```python
from build123d import *
from OCP.BRepFilletAPI import BRepFilletAPI_MakeChamfer

# Parameters (mm, degrees)
BOSS_EXTRUDE1_DEPTH        = 4
FILLET1_R                  = 2
FILLET2_R                  = 4
SKETCH3_R                  = 6
CUT_EXTRUDE3_DEPTH         = 61.942595941
SKETCH4_R                  = 1.75
CUT_EXTRUDE6_DEPTH         = 61.942595941
CUT_EXTRUDE7_DEPTH         = 10
CUT_EXTRUDE8_START         = -12.533
CUT_EXTRUDE8_DEPTH         = 25.3653
CHAMFER1_SIZE              = 2
CHAMFER1_SIZE_2            = 0.932615316
CHAMFER1_OF_MIRROR1_SIZE   = 0.932615316
CHAMFER1_OF_MIRROR1_SIZE_2 = 2
CHAMFER2_SIZE              = 0.5


with BuildPart() as part:
    # Sketch1 → Boss-Extrude1 (new body)
    with BuildSketch(Plane.XY):
        Polygon((43, -43), (43, 7), (35, 7), (35, 1), (-1, 1), (-1, -35), (-7, -35), (-7, -43), align=None)
    extrude(amount=BOSS_EXTRUDE1_DEPTH)

    # Fillet1
    fillet1_edges = [part.edges().sort_by_distance(p)[0] for p in [
        (-7, -43, 2),
        (-7, -35, 2),
        (-1, 1, 2),
        (35, 7, 2),
        (43, 7, 2),
        (43, -43, 2),
    ]]
    fillet(fillet1_edges, radius=FILLET1_R)

    # Fillet2
    fillet2_edges = [part.edges().sort_by_distance(p)[0] for p in [
        (35, 1, 2),
        (-1, -35, 2),
    ]]
    fillet(fillet2_edges, radius=FILLET2_R - 0.0001)  # a hair under: the kernel refuses the full size

    # Sketch3 → Cut-Extrude3 (cut, through all)
    with BuildSketch(Plane(origin=(0, 0, 0), x_dir=(-1, 0, 0), z_dir=(0, 0, -1))):
        with Locations((-17.899660586, -17.899660586)):
            Circle(SKETCH3_R)
    extrude(amount=-CUT_EXTRUDE3_DEPTH, mode=Mode.SUBTRACT)

    # Sketch4 → Cut-Extrude6 (cut, through all)
    with BuildSketch(Plane(origin=(0, 0, 0), x_dir=(-1, 0, 0), z_dir=(0, 0, -1))):
        with Locations((-39, 3)):
            Circle(SKETCH4_R)
        with Locations((-39, -39)):
            Circle(SKETCH4_R)
        with Locations((3, -39)):
            Circle(SKETCH4_R)
        with Locations((-2.025269256, -2.025269256)):
            Circle(SKETCH4_R)
    extrude(amount=-CUT_EXTRUDE6_DEPTH, mode=Mode.SUBTRACT)

    # Sketch5 → Cut-Extrude7 (cut, symmetric)
    with BuildSketch(Plane.ZY.offset(-17.899660586)):
        Polygon((2, -43), (0, -43), (0, -41), align=None)
    cut_extrude7 = extrude(amount=CUT_EXTRUDE7_DEPTH, both=True, mode=Mode.SUBTRACT)

    # Sketch6 → Cut-Extrude8 (cut)
    with BuildSketch(Plane.ZY.offset(-17.899660586).offset(CUT_EXTRUDE8_START)):
        Polygon((0, 1), (0, -1), (1.5, -1), (3.5, 1), align=None)
    cut_extrude8 = extrude(amount=CUT_EXTRUDE8_DEPTH, mode=Mode.SUBTRACT)

    # Chamfer1
    chamfer1_edges_1 = [part.edges().sort_by_distance(p)[0] for p in [
        (5.067360586, -1, 0.75),
    ]]
    chamfer1_side_1 = [part.faces().sort_by_distance(p)[0] for p in [
        (5.067360586, -0.981347694, 0.75),
    ]]
    chamfer1_edges_2 = [part.edges().sort_by_distance(p)[0] for p in [
        (30.432660586, -1, 0.75),
    ]]
    chamfer1_side_2 = [part.faces().sort_by_distance(p)[0] for p in [
        (30.41400828, -1, 0.75),
    ]]
    chamfer1 = BRepFilletAPI_MakeChamfer(part.part.solid().wrapped)
    for e in chamfer1_edges_1:
        chamfer1.Add(CHAMFER1_SIZE - 0.0001, CHAMFER1_SIZE_2 - 0.0001, e.wrapped, chamfer1_side_1[0].wrapped)
    for e in chamfer1_edges_2:
        chamfer1.Add(CHAMFER1_SIZE_2 - 0.0001, CHAMFER1_SIZE - 0.0001, e.wrapped, chamfer1_side_2[0].wrapped)
    add(Compound.cast(chamfer1.Shape()), mode=Mode.REPLACE)  # a hair under: the kernel refuses the full size

    # Mirror1: Cut-Extrude7, Cut-Extrude8 across plane
    add(cut_extrude7.mirror(Plane(origin=(0, 0, 0), x_dir=(0, 0, 1), z_dir=(-0.7071067811865479, -0.7071067811865472, 0))), mode=Mode.SUBTRACT)
    add(cut_extrude8.mirror(Plane(origin=(0, 0, 0), x_dir=(0, 0, 1), z_dir=(-0.7071067811865479, -0.7071067811865472, 0))), mode=Mode.SUBTRACT)

    # Chamfer1 of Mirror1
    chamfer1_of_mirror1_edges_1 = [part.edges().sort_by_distance(p)[0] for p in [
        (1, -5.067360586, 0.75),
    ]]
    chamfer1_of_mirror1_side_1 = [part.faces().sort_by_distance(p)[0] for p in [
        (1, -5.086012893, 0.75),
    ]]
    chamfer1_of_mirror1_edges_2 = [part.edges().sort_by_distance(p)[0] for p in [
        (1, -30.432660586, 0.75),
    ]]
    chamfer1_of_mirror1_side_2 = [part.faces().sort_by_distance(p)[0] for p in [
        (0.981347694, -30.432660586, 0.75),
    ]]
    chamfer1_of_mirror1 = BRepFilletAPI_MakeChamfer(part.part.solid().wrapped)
    for e in chamfer1_of_mirror1_edges_1:
        chamfer1_of_mirror1.Add(CHAMFER1_OF_MIRROR1_SIZE - 0.0001, CHAMFER1_OF_MIRROR1_SIZE_2 - 0.0001, e.wrapped, chamfer1_of_mirror1_side_1[0].wrapped)
    for e in chamfer1_of_mirror1_edges_2:
        chamfer1_of_mirror1.Add(CHAMFER1_OF_MIRROR1_SIZE_2 - 0.0001, CHAMFER1_OF_MIRROR1_SIZE - 0.0001, e.wrapped, chamfer1_of_mirror1_side_2[0].wrapped)
    add(Compound.cast(chamfer1_of_mirror1.Shape()), mode=Mode.REPLACE)  # a hair under: the kernel refuses the full size

    # Sketch7 → Revolve1 (revolve)
    with BuildSketch(Plane(origin=(0, -17.899660586, 0), x_dir=(0, 0, -1), z_dir=(0, -1, 0))):
        Polygon((0, 23.899660586), (5, 21.01290924), (5, 18.899660586), (1.365063509, 18.899660586), (-0.8, 20.149660586), (-4, 20.149660586), (-4, 23.899660586), align=None)
    revolve(axis=Axis((17.899660586, -17.899660586, 0), (0, 0, -1)))

    # Chamfer2
    chamfer2_edges = [part.edges().sort_by_distance(p)[0] for p in [
        (15.649660586, -17.899660586, 4),
    ]]
    chamfer(chamfer2_edges, length=CHAMFER2_SIZE)


solid = part.part
```
Verification items for the finished model (mm, model axes). A direction names the side the tool comes from. Coordinates: 2 decimals unless noted, no trailing zeros. Write each loop counter-clockwise with the first axis right and the second up, starting at its lowest first coordinate (ties: lowest second). Pieces come first, ordered by that corner, then holes. Notation, with made-up numbers: M 63.5,12 L 117.5,12 A5 cw 117.5,20 Z; hole C 55,-33.5 d3. An arc over 180 degrees is marked long. One line per item, written item: value.
Item 1: Section check D-D, the plane y = 3. Record the boundary of the cut face in (x, z), plus the area to 3 significant figures.
Check sheet entries:
outline: M 34.46,0 L 37.25,0 L 37.25,4 L 34.46,4 Z; M 40.75,0 L 43,0 L 43,4 L 40.75,4 Z
area: 20.1 mm^2
Item 2: Section check A-A, the plane x = 39. Record the boundary of the cut face in (y, z).
Check sheet entries:
outline: M -43,0 L -40.75,0 L -40.75,4 L -43,4 Z; M -37.25,0 L 1.25,0 L 1.25,4 L -37.25,4 Z; M 4.75,0 L 7,0 L 7,4 L 4.75,4 Z
Item 3: Scan lines: line 1 along Y through (x, z) = (39, 2.95); line 2 along X through (y, z) = (-39.5, 2.5); line 3 along Z through (x, y) = (33, -6). Record each from-to range of solid material in increasing order.
Check sheet entries:
line 1: y = -43 to -40.75, -37.25 to 1.25, 4.75 to 7
line 2: x = -7 to -4.68, -1.32 to 37.32, 40.68 to 43
line 3: z = 0 to 4
Item 4: Section check B-B, the plane y = -39. Record the boundary of the cut face in (x, z), plus the area to 3 significant figures.
Check sheet entries:
outline: M -7,0 L -4.75,0 L -4.75,4 L -7,4 Z; M -1.25,0 L 37.25,0 L 37.25,4 L -1.25,4 Z; M 40.75,0 L 43,0 L 43,4 L 40.75,4 Z
area: 172 mm^2
Item 5: Access from +Z, -Z, +X, -X, +Y, -Y to the whole of each face (thin tool, end or side, straight path). Record for faces 5 (the flat face through (27.9, -42.4, 0.6)), 6 (the flat face through (1, -18, 1)), 7 (the flat face through (-1, -9.3, 3.8)), 8 (the flat face through (5.437, 0.208, 1.337)).
Check sheet entries:
face 5: -Z, -Y
face 6: -Z, -X
face 7: +Z, -Z, -X, +Y
face 8: -Z, +Y
Item 6: Section check C-C, the plane x = 25.5. Record the boundary of the cut face in (y, z), plus the area to 3 significant figures.
Check sheet entries:
outline: M -43,2 L -41,0 L -1,0 L -1,1.5 L 1,3.5 L 1,4 L -43,4 Z
area: 169 mm^2
Item 7: Mould release check, pull along X, two halves, no side actions. Record for faces 1 (the flat face through (18, -42, 1)), 2 (the cylindrical face through (-2.62, -40.71, 1.97)), 3 (the cylindrical face through (-2.203, -33.859, 2.028)), 4 (the flat face through (23, -18, 4)): pulls with the +X half, pulls with the -X half, needs draft (parallel to the pull), parting line crosses it, or undercut.
Check sheet entries:
face 1: undercut
face 2: undercut
face 3: pulls with the -X half
face 4: needs draft
Item 8: Gauge pin test, flat ends, axial feed: pin 1 Ø1 at (y, z) = (-42, 1.5) entering from -X; pin 2 Ø2.5 at (x, y) = (17.9, -17.9) entering from +Z; pin 3 Ø4 at (x, y) = (30.5, -28) entering from -Z; pin 4 Ø10 at (x, y) = (9, 1.5) entering from +Z. Record the tip position at first contact, or that the pin passes through.
Check sheet entries:
pin 1: stops at x = -6.94
pin 2: stops at z = -0.93
pin 3: stops at z = 0
pin 4: stops at z = 4
